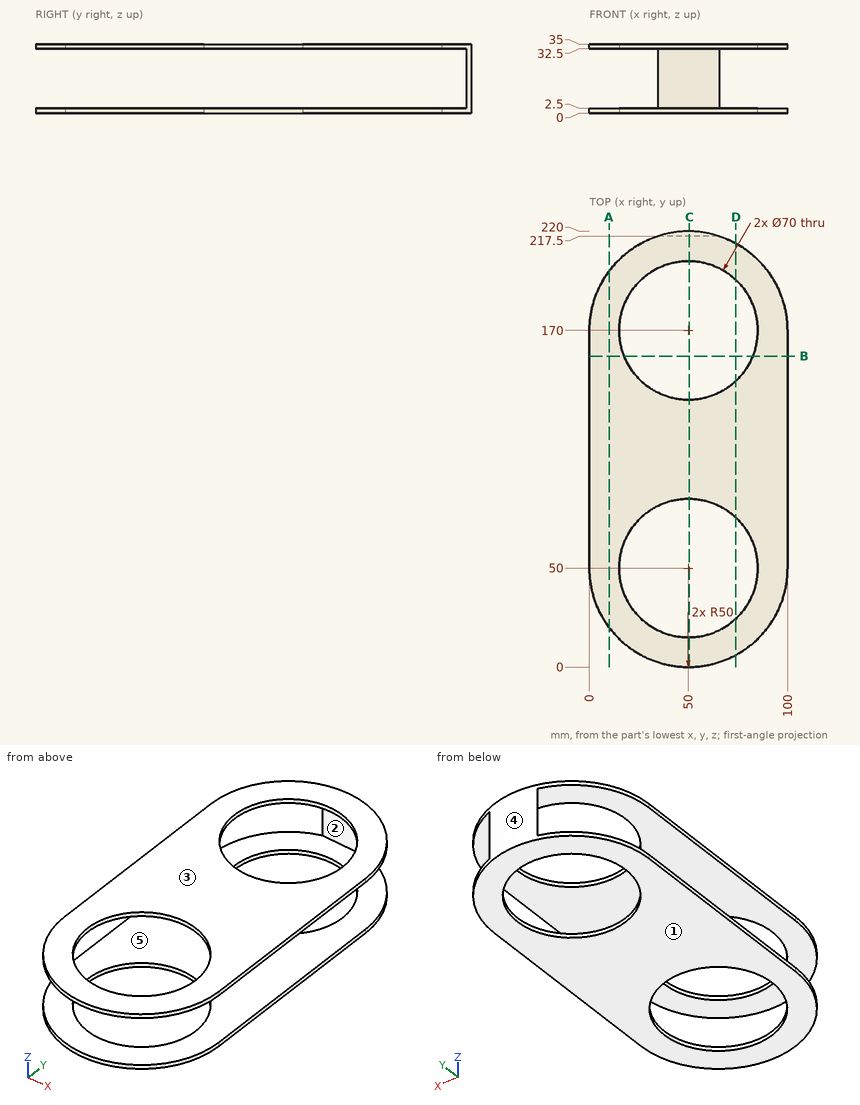
Verification items for this drawing (mm, ordinates from the low corner). A direction names the side the tool comes from. Give positions to 0.01 mm unless a question says otherwise; leave off trailing zeros. Loops run counter-clockwise (first coordinate to the right, second up) from the corner with the lowest first, then second, coordinate; pieces in that order, holes last.
(1) Section check A-A on x = 10. Record the cut outline in (y, z), then the cut area to 3 significant figures.
From the geometry:
outline: (20, 0) - (200, 0) - (200, 2.5) - (20, 2.5) - close; (20, 32.5) - (200, 32.5) - (200, 35) - (20, 35) - close
area: 900 mm2
(2) Set-up check for the marked faces 4 and 5: record each of +Z, -Z, +X, -X, +Y, -Y from which the full face is reachable in a straight line by a thin tool's end or side.
From the geometry:
face 4: +Z, -Z, +Y
face 5: +X, -X, -Y
(3) Section check D-D on x = 74. Record the cut outline in (y, z).
From the geometry:
outline: (6.14, 0) - (24.52, 0) - (24.52, 2.5) - (6.14, 2.5) - close; (6.14, 32.5) - (24.52, 32.5) - (24.52, 35) - (6.14, 35) - close; (75.48, 0) - (144.52, 0) - (144.52, 2.5) - (75.48, 2.5) - close; (75.48, 32.5) - (144.52, 32.5) - (144.52, 35) - (75.48, 35) - close; (195.48, 0) - (213.86, 0) - (213.86, 2.5) - (195.48, 2.5) - close; (195.48, 32.5) - (213.86, 32.5) - (213.86, 35) - (195.48, 35) - close
(4) Thickness scan on L1, parallel to Y at x = 50, z = 33.55; L2, parallel to Z at x = 63, y = 117.5; L3, parallel to X at y = 170, z = 34.3. Record the ranges inside material, lowest first.
From the geometry:
L1: y = 0 to 15, 85 to 135, 205 to 220
L2: z = 0 to 2.5, 32.5 to 35
L3: x = 0 to 15, 85 to 100
(5) Section check B-B on y = 157. Record the cut outline in (x, z).
From the geometry:
outline: (0, 0) - (17.5, 0) - (17.5, 2.5) - (0, 2.5) - close; (0, 32.5) - (17.5, 32.5) - (17.5, 35) - (0, 35) - close; (82.5, 0) - (100, 0) - (100, 2.5) - (82.5, 2.5) - close; (82.5, 32.5) - (100, 32.5) - (100, 35) - (82.5, 35) - close
(6) Section check C-C on x = 50.5. Record the cut outline in (y, z), then the cut area to 3 significant figures.
From the geometry:
outline: (0, 0) - (15, 0) - (15, 2.5) - (0, 2.5) - close; (0, 32.5) - (15, 32.5) - (15, 35) - (0, 35) - close; (85, 0) - (135, 0) - (135, 2.5) - (85, 2.5) - close; (85, 32.5) - (135, 32.5) - (135, 35) - (85, 35) - close; (205, 0) - (220, 0) - (220, 35) - (205, 35) - (205, 32.5) - (217.5, 32.5) - (217.5, 2.5) - (205, 2.5) - close
area: 475 mm2
(7) Depth check by flat-ended pin: pin 1 Ø8 at (x, z) = (47.5, 9) entering from +Y; pin 2 Ø10 at (x, z) = (32.5, 8.5) entering from +Y; pin 3 Ø5 at (x, z) = (32, 11) entering from +Y. Enter the tip coordinate at first touch or a pass-through.
From the geometry:
pin 1: stops at y = 220
pin 2: stops at y = 218.41
pin 3: stops at y = 217.54
(8) Release check for a two-part mould opening along Z. For the marked faces 1, 2 and 3 record: released by +Z, released by -Z, zero draft, split by the parting line, or undercut.
From the geometry:
face 1: released by -Z
face 2: undercut
face 3: released by +Z
